Part model, mm, in its own coordinate system. A direction names the side the tool comes from. Give positions to 0.01 mm unless a question says otherwise; leave off trailing zeros. Use a Markdown table: item, result. Add a question column.
Autodesk Fusion 360 part; units mm, degrees
sketch "Sketch1" plane through (0, 0, 0) normal (0, 1, 0) x (1, 0, 0)
  line L0 (0, 0) -> (-15, 0)
  line L1 (0, 0) -> (15, 0)
  circle A0 centre (15, 0) radius 3
  circle A1 centre (-15, 0) radius 3
  circle A2 centre (15, 0) radius 4
  circle A3 centre (-15, 0) radius 4
  circle A4 centre (0, 0) radius 11
  circle A5 centre (0, 0) radius 19
  line L2 (0, 0) -> (0, -15)
  line L3 (0, 0) -> (0, 15)
  line L4 (0, -15) -> (20.2663, -15)
  line L5 (20.2663, -15) -> (-18, -15)
  line L6 (0, 15) -> (-22, 15)
  line L7 (-22, 15) -> (21.8454, 15.4076)
  dimension "d1" = 15
  dimension "d2" = 15
  dimension "d3" = 6
  dimension "d4" = 6
  dimension "d5" = 8
  dimension "d6" = 8
  dimension "d7" = 38
  dimension "d8" = 15
  dimension "d9" = 15
extrude "Extrude1" add sketch "Sketch1" along normal blind 5 contours A1 | A3 | A3 A4 A5 L2 L5 | A3 A4 A5 L3 L6 | A0 | A2 A4 A5 L3 L6 L7 | A2 | A2 A4 A5 L2 L4 L5
extrude "Extrude2" cut sketch "Sketch1" along normal blind 3.7 contours A1 | A0
fillet "Fillet1" radius 2 2 faces at (16.9556, 3.7, 0.2948) (-15.2176, 3.7, -0.9086)
fillet "Fillet2" radius 1 2 edges at (12.203, 0, 1.0848) (-17.797, 0, 1.0848)
fillet "Fillet3" radius 2 4 edges at (-11.6619, 2.5, 15) (11.6619, 2.5, 15) (-11.5357, 2.5, -15.0973) (11.253, 2.5, -15.3091)
fillet "Fillet4" radius 1 1 faces at (-0.3682, 5, -13.7919)
1. Drill centre lines: probe 1 along X at (y, z) = (1.25, 0); probe 2 along Z at (x, y) = (-15.5, 2.15); probe 3 along Z at (x, y) = (-15, 1.1). Where is each one in solid material? Low to high. Write a range as [from, to].
2. Tool access for faces 4 (the cylindrical face through (0.01, 4.7, -14.92)), 5 (the cylindrical face through (-19, 2, 0)), 6 (the cylindrical face through (12, 1.3, 0.1)): list every direction of +Z, -Z, +X, -X, +Y, -Y with a clear straight run to the whole face (end or side of a thin tool).
3. Cut at A-A (y = 2.65). Give the number of separate pieces and of enclosed holes in the cut face, then the cut area to 3 significant figures.
4. Flat gauge pins, fed straight in: pin 1 (2 mm diameter, centred on y = 1, z = -11, fed in from +X); pin 2 (3 mm diameter, centred on x = 4, z = 9.5, fed in from +Y); pin 3 (1.6 mm diameter, centred on x = 15.5, z = 0, fed in from -Y). Where does each tip first touch, or does it go through?
5. Mould opens along X. For faces 1 (the flat face through (0, 2, 15)), 2 (the cylindrical face through (-11.65, 2.028, 14.875)), 3 (the cylindrical face through (-18, 1.3, 0.1)) say: released by +X, released by -X, zero draft, split by the parting line, or undercut.
A:
| question | item | result |
|---|---|---|
| 1 | probe 1 | x = [-19, -18], [-12, -11], [11, 12], [18, 19] |
| 1 | probe 2 | z = [-10.99, -2.91], [2.91, 10.99] |
| 1 | probe 3 | z = [-11.66, -3], [3, 11.66] |
| 2 | face 4 | -Z, -X, +Y |
| 2 | face 5 | -X, +Y, -Y |
| 2 | face 6 | -Y |
| 3 | separate pieces | 1 |
| 3 | enclosed holes | 3 |
| 3 | area | 583 mm² |
| 4 | pin 1 | stops at x = 16.16 |
| 4 | pin 2 | stops at y = 4.98 |
| 4 | pin 3 | stops at y = 3.68 |
| 5 | face 1 | zero draft |
| 5 | face 2 | released by -X |
| 5 | face 3 | undercut |
